Model file for the job. Use its own axes, mm. Coordinates: 2 decimals unless noted, no trailing zeros. Write each loop counter-clockwise with the first axis right and the second up, starting at its lowest first coordinate (ties: lowest second). Pieces come first, ordered by that corner, then holes. Notation, with made-up numbers: M -27,77.25 L -12,77.25 A31 cw -12,109.25 Z; hole C -8,50.5 d6. An arc over 180 degrees is marked long. One line per question, with ' | ' between items. Start each with the question number.
(1) Flat gauge pins, fed straight in: pin 1 Ø6 at (y, z) = (5.5, 3.5) entering from +X; pin 2 Ø1 at (y, z) = (-34, -1.5) entering from +X; pin 3 Ø6 at (x, y) = (-2, -182.5) entering from +Z; pin 4 Ø6 at (x, z) = (-0.5, 32) entering from +Y. Where does each tip first touch, or does it go through?
(2) Wall check: probe 1 along Z at (x, y) = (0, -92); probe 2 along X at (y, z) = (-53.5, 18); probe 3 along Z at (x, y) = (2.75, -303). Give the ranges that are in metal, low to high.
(3) Cut at B-B (y = -5). Write the cut outline in (x, z).
(4) Cut at A-A (x = 0). Write the cut outline in (y, z), plus the area to 3 significant figures.
(5) Cut at C-C (z = 28.5). Write the cut outline in (x, y).
from build123d import *

# Parameters (mm, degrees)
F0_R     = 4.826
F1_DEPTH = 381


with BuildPart() as f1:
    # F0 (on Front) → F1 (new body, symmetric)
    with BuildSketch(Plane.XZ):
        with BuildLine():
            Line((-8.001, 50.8), (-8.001, 0))
            ThreePointArc((-8.001, 0), (0, -8.001), (8.001, 0))
            ThreePointArc((8.001, 0), (3.563929, 7.163408), (-4.826, 6.381671))
            Line((-4.826, 6.381671), (-4.826, 50.8))
            Line((-4.826, 50.8), (-8.001, 50.8))
        make_face()
        Circle(F0_R, mode=Mode.SUBTRACT)
    extrude(amount=F1_DEPTH, both=True)


solid = f1.part
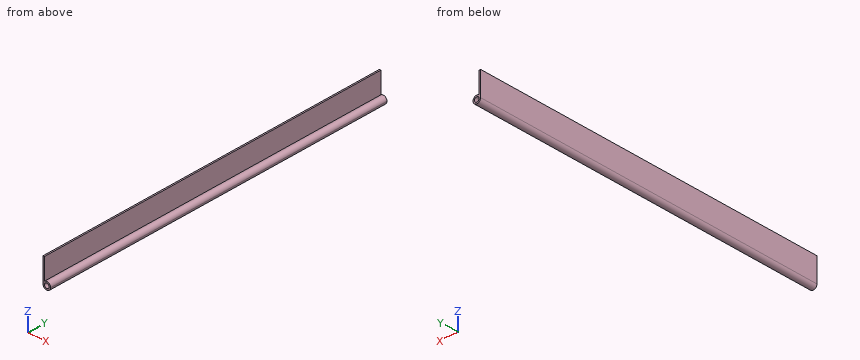
Filled in:
1) pin 1: x = 7.99 | pin 2: x = 7.94 | pin 3: z = 50.8 | pin 4: through
2) probe 1: -8 to -4.83, 4.83 to 8 | probe 2: -8 to -4.83 | probe 3: -7.51 to -3.97, 3.97 to 7.51
3) outline: M -8,0 A8 ccw long -4.83,6.38 L -4.83,50.8 L -8,50.8 Z; hole C 0,0 d9.65
4) outline: M -381,-8 L 381,-8 L 381,-4.83 L -381,-4.83 Z; M -381,4.83 L 381,4.83 L 381,8 L -381,8 Z | area: 4,840 mm²
5) outline: M -8,-381 L -4.83,-381 L -4.83,381 L -8,381 Z
